from build123d import *

# Parameters (mm, degrees)
SKETCH1_W                       = 323.85
SKETCH1_H                       = 222.25
BOSS_EXTRUDE1_DEPTH             = 3.175
M5_CLEARANCE_HOLE1_D            = 5.5
F_9_64_0_14063_DIAMETER_HOLE1_D = 3.572002


with BuildPart() as part:
    # Sketch1 → Boss-Extrude1 (new, symmetric)
    with BuildSketch(Plane(origin=(0, 0, 0), x_dir=(1, 0, 0), z_dir=(0, 1, 0))):
        Rectangle(SKETCH1_W, SKETCH1_H)
    extrude(amount=BOSS_EXTRUDE1_DEPTH, both=True)

    # M5 Clearance Hole1 (through all)
    with Locations(Plane(origin=(0, 3.175, 0), x_dir=(1, 0, 0), z_dir=(0, 1, 0))):
        with Locations((-144.399, 94.3991), (144.399, 94.3991), (144.399, -94.3991), (-144.399, -94.3991)):
            Hole(M5_CLEARANCE_HOLE1_D / 2)

    # 9/64 (0.14063) Diameter Hole1 (through all)
    with Locations(Plane(origin=(0, 3.175, 0), x_dir=(1, 0, 0), z_dir=(0, 1, 0))):
        with Locations((-149.225, 60.325), (-149.225, -47.625), (136.525, 60.325), (136.525, -47.625)):
            Hole(F_9_64_0_14063_DIAMETER_HOLE1_D / 2)


solid = part.part
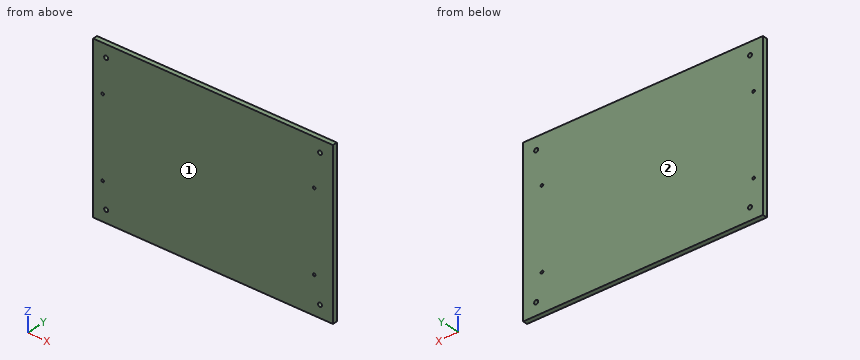
Verification items for the finished model (mm, model axes). Face numbers are marked on the shaded views. Round coordinates to 2 decimals unless told otherwise and drop trailing zeros. Put each result on its own line as item: value.
1) Depth check by flat-ended pin: pin 1 (4.5 mm diameter, centred on x = 144.4, z = 94.4, fed in from -Y). Enter the tip coordinate at first touch or a pass-through.
Final values:
pin 1: passes through
2) Mould release check, pull along Y, two halves, no side actions. Record for the marked faces 1 and 2: +Y half, -Y half, draft (parallel to the pull), parting line (faces both ways), or undercut.
Final values:
face 1: -Y half
face 2: +Y half
3) Material ranges on line 1 (Z direction, x = 144, y = 1.75) (3 decimals); line 2 (Z direction, x = 137, y = 1.5) (3 decimals); line 3 (X direction, y = 1.75, z = -96) (3 decimals), recorded low to high.
Final values:
line 1: z = -111.125 to -97.12, -91.678 to 91.678, 97.12 to 111.125
line 2: z = -111.125 to -62.047, -58.603 to 45.903, 49.347 to 111.125
line 3: x = -161.925 to -146.635, -142.163 to 142.163, 146.635 to 161.925
